Source: three-view drawing plus pictorial views. Frame: mm from the lowest corner of the part. A direction names the side the tool comes from. Give positions to 0.01 mm unless a question says otherwise; leave off trailing zeros. Loops run counter-clockwise (first coordinate to the right, second up) from the corner with the lowest first, then second, coordinate; pieces in that order, holes last. Notation, with made-up numbers: (52.5, -23.75) - (77.5, -23.75) arc R18 ccw to (77.5, -3.75) - close; hole circle Ø8 at (-36, -8.75). An arc over 180 degrees is marked (long way). One line per item, written item: value.
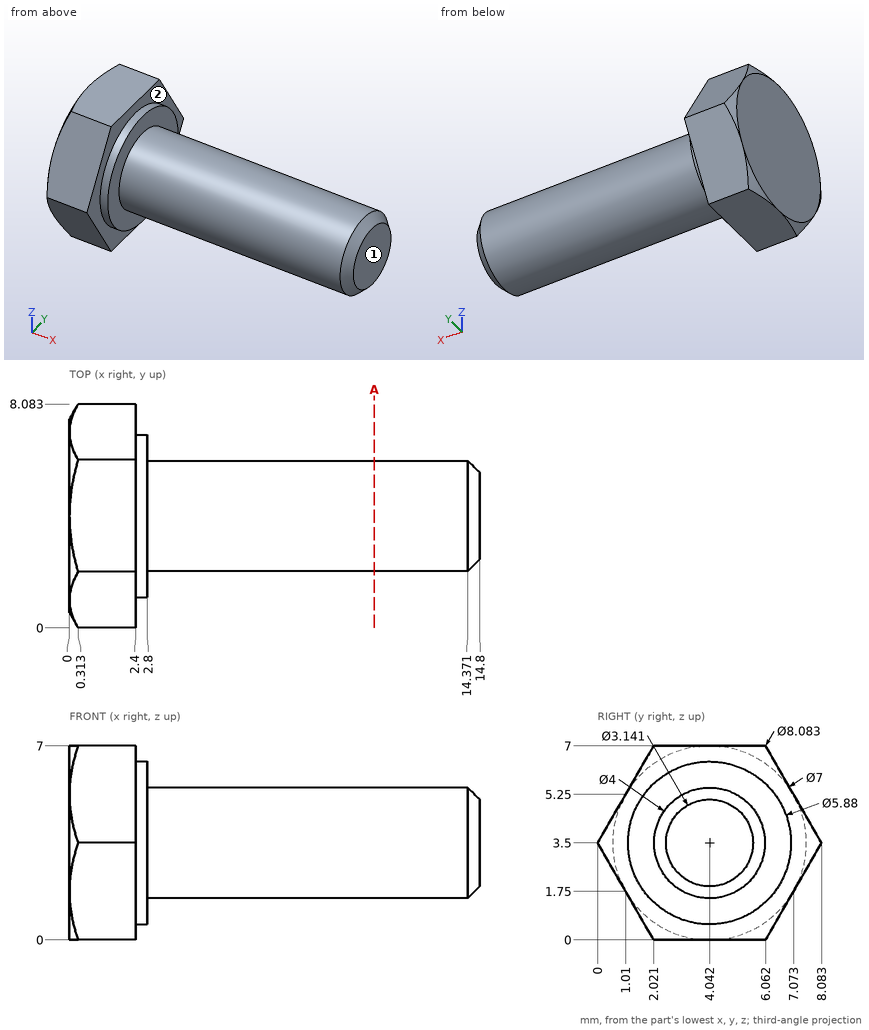
Item 1: Section A-A, the plane x = 11. Output: boundary loops of the cut face in (y, z).
Verdict:
outline: circle Ø4 at (4.04, 3.5)
Item 2: Access query for the marked faces 1 and 2. Directions: +Z, -Z, +X, -X, +Y, -Y. A direction counts if a zero-diameter tool reaches every point of the face in a straight line with its end or side. Return the directions, or none.
Verdict:
face 1: +Z, -Z, +X, +Y, -Y
face 2: +X
Item 3: Material intervals for L1, parallel to X at y = 7.5, z = 3; L2, parallel to X at y = 6.25, z = 5; L3, parallel to Z at x = 8.75, y = 4, sorted ascending.
Verdict:
L1: x = 0 to 2.4
L2: x = 0 to 2.8
L3: z = 1.5 to 5.5
